Geometry: final body of the model. Coordinates: model frame, mm. A direction names the side the tool comes from. Coordinates: 2 decimals unless noted, no trailing zeros. Order: outer loops, then holes, each group sorted by start corner. A loop starts at its lowest first (then second) coordinate and runs counter-clockwise, first axis right, second up. Notation, with made-up numbers: (-29.75, 9.25) -> (-6.75, 9.25) arc R23 ccw to (-6.75, 22.25) -> close; hole circle Ø8 at (-38.5, 29). An arc over 180 degrees is marked (long way). Answer in a Markdown table with one row per item. Add a question column.
1) Section query B-B on x = 13.5. Return the cut outline in (y, z).
2) Pull-direction query (X, two-part tool) for faces 5 (the face through (10, 0, -25)), 6 (the face through (4, 3, -27)), 7 (the face through (20, 5, -25)), 8 (the face through (13, 3, -36)); classes: +X half, -X half, draft (parallel to the pull), parting line (faces both ways), or undercut.
3) Section query C-C on y = 0.8. Count the separate pieces of the cut face and the enclosed holes in it, then the cut area to 3 significant figures.
4) Contact query for flat-ended pins moving along their axis: P1, Ø1, axis at x = 17.5, z = -17, coming from the -Y side; P2, Ø4, axis at x = 6, z = -36, coming from the -Y side. Output: stop coordinate, or through.
5) Set-up query: faces 1 (the face through (14, 3, -29)), 2 (the face through (18, 2, -27.6)), 3 (the face through (4.659, 1.479, -29.233)), 4 (the face through (10, 6, -25)). Return all of +Z, -Z, +X, -X, +Y, -Y with unobstructed straight access to the full face (end or side cutting, diameter ignored); none if empty.
6) Section query A-A on z = -26. Return the cut outline in (x, y), then the cut area to 3 significant figures.
7) Ray query, line 1 (Z direction, x = 13.75, y = 1.85); line 2 (Z direction, x = 18, y = 1.4); line 3 (X direction, y = 2.05, z = -34). Return the intervals inside material, ascending. Write a range as from..to.
8) Section query D-D on x = 6. Return the cut outline in (y, z), then the cut area to 3 significant figures.
```python
from build123d import *

# Parameters (mm, degrees)
SKETCH_1_W          = 20
SKETCH_1_H          = 50
EXTRUDE_1_DEPTH     = 6
SKETCH_3_W          = 4
SKETCH_3_H          = 3.2
CUT_EXTRUDE_1_DEPTH = 4.5
SKETCH_5_R          = 1.6
SKETCH_5_W          = 3
SKETCH_5_H          = 6
CUT_EXTRUDE_2_DEPTH = 14.5
SKETCH_7_R          = 3.5
CUT_EXTRUDE_3_DEPTH = 3


with BuildPart() as part:
    # 草图1 → 凸台-拉伸1 (new body)
    with BuildSketch(Plane(origin=(0, 0, 0), x_dir=(1, 0, 0), z_dir=(0, 1, 0))):
        with Locations((10, 25)):
            Rectangle(SKETCH_1_W, SKETCH_1_H)
    extrude(amount=EXTRUDE_1_DEPTH)

    # 草图3 → 切除-拉伸1 (cut)
    with BuildSketch(Plane.XZ):
        with Locations((18, -26)):
            Rectangle(SKETCH_3_W, SKETCH_3_H)
        with Locations((18, -16)):
            Rectangle(SKETCH_3_W, SKETCH_3_H)
        with Locations((18, -36)):
            Rectangle(SKETCH_3_W, SKETCH_3_H)
    extrude(amount=-CUT_EXTRUDE_1_DEPTH, mode=Mode.SUBTRACT)

    # 草图5 → 切除-拉伸2 (cut)
    with BuildSketch(Plane.XZ):
        with Locations(Location((6, -16, 0), (0, 0, 270))):
            Circle(SKETCH_5_R)
        with Locations(Location((6, -26, 0), (0, 0, 270))):
            Circle(SKETCH_5_R)
        with Locations(Location((6, -36, 0), (0, 0, 270))):
            Circle(SKETCH_5_R)
        with Locations((14.5, -36)):
            Rectangle(SKETCH_5_W, SKETCH_5_H)
        with Locations((14.5, -26)):
            Rectangle(SKETCH_5_W, SKETCH_5_H)
        with Locations((14.5, -16)):
            Rectangle(SKETCH_5_W, SKETCH_5_H)
    extrude(amount=-CUT_EXTRUDE_2_DEPTH, mode=Mode.SUBTRACT)

    # 草图7 → 切除-拉伸3 (cut)
    with BuildSketch(Plane.XZ):
        with Locations(Location((6, -16, 0), (0, 0, 270))):
            Circle(SKETCH_7_R)
        with Locations(Location((6, -26, 0), (0, 0, 270))):
            Circle(SKETCH_7_R)
        with Locations(Location((6, -36, 0), (0, 0, 270))):
            Circle(SKETCH_7_R)
    extrude(amount=-CUT_EXTRUDE_3_DEPTH, mode=Mode.SUBTRACT)


solid = part.part
```
Result:
| question | item | result |
|---|---|---|
| 1 | outline | (0, -50) -> (6, -50) -> (6, -39) -> (0, -39) -> close; (0, -33) -> (6, -33) -> (6, -29) -> (0, -29) -> close; (0, -23) -> (6, -23) -> (6, -19) -> (0, -19) -> close; (0, -13) -> (6, -13) -> (6, 0) -> (0, 0) -> close |
| 2 | face 5 | draft |
| 2 | face 6 | undercut |
| 2 | face 7 | +X half |
| 2 | face 8 | undercut |
| 3 | separate pieces | 1 |
| 3 | enclosed holes | 3 |
| 3 | area | 792 mm2 |
| 4 | P1 | y = 4.5 |
| 4 | P2 | y = 3 |
| 5 | face 1 | +Y, -Y |
| 5 | face 2 | +X, -Y |
| 5 | face 3 | -Y |
| 5 | face 4 | +Z, -Z, +X, -X, +Y |
| 6 | outline | (0, 0) -> (2.5, 0) -> (2.5, 3) -> (4.4, 3) -> (4.4, 6) -> (0, 6) -> close; (7.6, 3) -> (9.5, 3) -> (9.5, 0) -> (13, 0) -> (13, 6) -> (7.6, 6) -> close; (16, 4.5) -> (20, 4.5) -> (20, 6) -> (16, 6) -> close |
| 6 | area | 53.4 mm2 |
| 7 | line 1 | -50..-39, -33..-29, -23..-19, -13..0 |
| 7 | line 2 | -50..-37.6, -34.4..-27.6, -24.4..-17.6, -14.4..0 |
| 7 | line 3 | 0..3.13, 8.87..13, 16..20 |
| 8 | outline | (0, -50) -> (6, -50) -> (6, -37.6) -> (3, -37.6) -> (3, -39.5) -> (0, -39.5) -> close; (0, -32.5) -> (3, -32.5) -> (3, -34.4) -> (6, -34.4) -> (6, -27.6) -> (3, -27.6) -> (3, -29.5) -> (0, -29.5) -> close; (0, -22.5) -> (3, -22.5) -> (3, -24.4) -> (6, -24.4) -> (6, -17.6) -> (3, -17.6) -> (3, -19.5) -> (0, -19.5) -> close; (0, -12.5) -> (3, -12.5) -> (3, -14.4) -> (6, -14.4) -> (6, 0) -> (0, 0) -> close |
| 8 | area | 208 mm2 |
